Geometry: final body of the model. Coordinates: model frame, mm. A direction names the side the tool comes from. Give positions to 0.01 mm unless a question says otherwise; leave off trailing zeros. Write each loop counter-clockwise with the first axis right and the second up, starting at its lowest first coordinate (ties: lowest second). Pieces come first, ordered by that corner, then holes. Notation, with made-up numbers: (61.25, 2.25) -> (65.25, 2.25) arc R30 cw to (65.25, 29.25) -> close; hole circle Ø6 at (77.5, -9). An arc over 180 degrees is marked (long way). Answer in a Markdown table with one row per item. Add a question column.
Item 1: Section query C-C on y = -18.5. Output: boundary loops of the cut face in (x, z), plus the area to 3 significant figures.
Item 2: First-contact query: P1, Ø1.5, axis at x = 1.5, y = -18.5, coming from the +Z side; P2, Ø1, axis at x = 4, z = 11, coming from the +Y side; P3, Ø1.5, axis at x = 1.5, y = 2.5, coming from the -Z side. Flat tips, straight axial feed; report the tip coordinate or a pass-through.
Item 3: Material intervals for probe 1 along Z at (x, y) = (4.05, -17); probe 2 along Y at (x, z) = (0.9, 14); probe 3 along Z at (x, y) = (0.9, -27), sorted ascending. Write a range as from..to.
Item 4: Access query for faces 1 (the flat face through (2, -25.417, -13)), 2 (the flat face through (2, -34.385, -8)), 3 (the flat face through (2, -8, 36.165)). Directions: +Z, -Z, +X, -X, +Y, -Y. A direction counts if a zero-diameter tool reaches every point of the face in a straight line with its end or side. Return the directions, or none.
Item 5: Section query B-B on z = -23.5. Output: boundary loops of the cut face in (x, y), plus the area to 3 significant figures.
Item 6: Section query A-A on x = 2.05. Output: boundary loops of the cut face in (y, z).
Autodesk Inventor part; units mm, degrees
ref_plane "YZ Plane" through (0, 0, 0) normal (1, 0, 0) x (0, 1, 0)
ref_plane "XZ Plane" through (0, 0, 0) normal (0, 1, 0) x (-1, 0, 0)
ref_plane "XY Plane" through (0, 0, 0) normal (0, 0, 1) x (1, 0, 0)
sketch "Esquisse1" plane through (0, 0, 0) normal (1, 0, 0) x (0, 1, 0)
  circle A0 centre (0, 0) radius 22.5 construction
  line L0 (24.5829, 26.4096) -> (-25.4171, 26.4096)
  line L1 (-25.4171, 26.4096) -> (-25.4171, -53.5904)
  line L2 (24.5829, 26.4096) -> (39.9583, 94.7002)
  line L3 (39.9583, 94.7002) -> (29.9583, 94.7002)
  line L4 (29.9583, 94.7002) -> (16.7794, 36.1654)
  line L5 (16.7794, 36.1654) -> (-34.3848, 36.1654)
  line L6 (-34.3848, 36.1654) -> (-34.3848, -53.5904)
  line L7 (-34.3848, -53.5904) -> (-25.4171, -53.5904)
  dimension "d0" = 45
  dimension "d1" = 50
  dimension "d2" = 80
  dimension "d3" = 70
  dimension "d4" = 10
  dimension "d5" = 60
  dimension "d6" = 102.688
  dimension "d7" = 102.688
  dimension "d8" = 51.1642
extrude "Extrusion1" add sketch "Esquisse1" along normal blind 5
Findings below:
| question | item | result |
|---|---|---|
| 1 | outline | (0, 26.41) -> (5, 26.41) -> (5, 36.17) -> (0, 36.17) -> close |
| 1 | area | 48.8 mm^2 |
| 2 | P1 | stops at z = 36.17 |
| 2 | P2 | stops at y = -25.42 |
| 2 | P3 | stops at z = 26.41 |
| 3 | probe 1 | z = 26.41..36.17 |
| 3 | probe 2 | y = -34.38..-25.42 |
| 3 | probe 3 | z = -53.59..36.17 |
| 4 | face 1 | -Z, +X, -X, +Y |
| 4 | face 2 | +Z, -Z, +X, -X, -Y |
| 4 | face 3 | +Z, +X, -X, -Y |
| 5 | outline | (0, -34.38) -> (5, -34.38) -> (5, -25.42) -> (0, -25.42) -> close |
| 5 | area | 44.8 mm^2 |
| 6 | outline | (-34.38, -53.59) -> (-25.42, -53.59) -> (-25.42, 26.41) -> (24.58, 26.41) -> (39.96, 94.7) -> (29.96, 94.7) -> (16.78, 36.17) -> (-34.38, 36.17) -> close |
